Design review of the part built by this model. Coordinates are the model's own, in mm. Face numbers are marked on the shaded views. A direction names the side the tool comes from. Coordinates: 2 decimals unless noted, no trailing zeros. Order: outer loops, then holes, each group sorted by start corner. A loop starts at its lowest first (then second) coordinate and runs counter-clockwise, first axis right, second up. Notation, with made-up numbers: (30, 65.25) -> (87, 65.25) arc R17 ccw to (87, 75.25) -> close; hole circle Ø3 at (5.25, -36.75). An arc over 180 degrees is marked (long way). Write item = value, one per line.
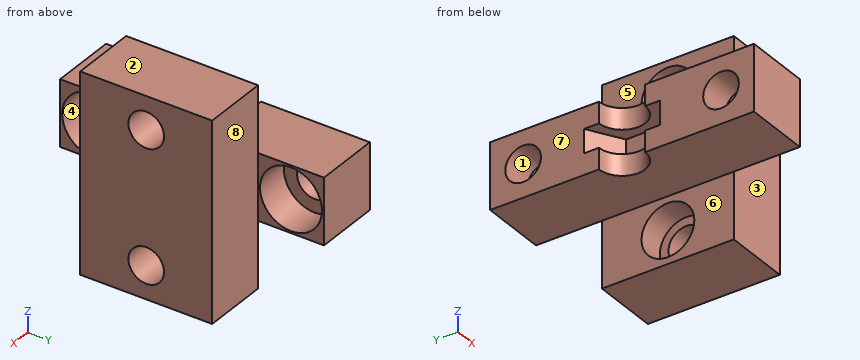
Autodesk Inventor part; units mm, degrees
ref_plane "YZ Plane" through (0, 0, 0) normal (1, 0, 0) x (0, 1, 0)
ref_plane "XZ Plane" through (0, 0, 0) normal (0, 1, 0) x (-1, 0, 0)
ref_plane "XY Plane" through (0, 0, 0) normal (0, 0, 1) x (1, 0, 0)
sketch "Sketch1" plane through (0, 0, 0) normal (0, 0, 1) x (1, 0, 0)
  line L0 (10, -10) -> (-10, -10)
  line L1 (-10, -10) -> (-10, 10)
  line L2 (-10, 10) -> (10, 10)
  line L3 (10, 10) -> (10, -10)
  line L4 (10, -10) -> (-10, 10) construction
  line L5 (-10, -10) -> (10, 10) construction
  line L6 (10, -10) -> (6, -10)
  line L7 (6, 10) -> (10, 10)
  line L8 (10, 10) -> (10, -10)
  line L9 (0, 10) -> (0, -10)
  line L10 (0, -10) -> (0, 10)
  point P0 (0, 0)
  dimension "d0" = 20
  dimension "d1" = 20
extrude "Extrusion1" add sketch "Sketch1" along normal blind 5 contours L0 L9 L2 L3
ref_plane "Work Plane1" through (0, 0, 2.5) normal (0, 0, 1) x (1, 0, 0)
sketch "Sketch2" plane through (0, 0, 2.5) normal (0, 0, 1) x (1, 0, 0)
  line L0 (0, 10) -> (0, -10)
  line L1 (0, 2.8868) -> (2.5, 1.4434)
  line L2 (2.5, 1.4434) -> (2.5, -1.4434)
  line L3 (2.5, -1.4434) -> (0, -2.8868)
  line L4 (0, -2.8868) -> (-2.5, -1.4434)
  line L5 (-2.5, -1.4434) -> (-2.5, 1.4434)
  line L6 (-2.5, 1.4434) -> (0, 2.8868)
  point P0 (0, 0)
  point P1 (0, 0)
  dimension "d12" = 5
extrude "Extrusion2" cut sketch "Sketch2" along normal mid plane 1.8
sketch "Sketch3" plane through (0, 0, 5) normal (0, 0, 1) x (1, 0, 0)
  circle A0 centre (0, 0) radius 1.75
  dimension "d15" = 3.5
extrude "Extrusion3" cut sketch "Sketch3" against normal blind 8
sketch "Sketch4" plane through (10, -10, 0) normal (1, 0, 0) x (0, 0, -1)
  circle A0 centre (-2.5, 17.5) radius 1.35
  circle A1 centre (-2.5, 2.5) radius 1.35
  line L0 (0, 20) -> (-5, 20)
  line L1 (0, 0) -> (-5, 0)
  line L2 (0, 0) -> (0, 20)
  point P0 (0, 10)
  dimension "d18" = 2.5
  dimension "d19" = 2.5
  dimension "d20" = 2.5
  dimension "d21" = 2.5
  dimension "d22" = 2.7
  dimension "d23" = 2.7
extrude "Extrusion4" cut sketch "Sketch4" against normal blind 25
sketch "Sketch5" plane through (10, -10, 0) normal (1, 0, 0) x (0, 0, -1)
  circle A0 centre (-2.5, 17.5) radius 1.35
  circle A1 centre (-2.5, 17.5) radius 2
  circle A2 centre (-2.5, 2.5) radius 1.35
  circle A3 centre (-2.5, 2.5) radius 2
  point P0 (0, 10)
  dimension "d26" = 4
  dimension "d27" = 4
extrude "Extrusion5" cut sketch "Sketch5" against normal blind 4 contours A0 | A1 | A2 | A3
sketch "Sketch6" plane through (0, 0, 5) normal (0, 0, 1) x (1, 0, 0)
  point P0 (0, 0)
sketch "Sketch7" plane through (0, 0, 5) normal (0, 0, 1) x (1, 0, 0)
  line L0 (10, -10) -> (10, 10)
  line L1 (10, 10) -> (5, 10)
  line L2 (5, 10) -> (5, 5)
  line L3 (5, 5) -> (10, 5)
  line L4 (10, 5) -> (10, 10)
  line L5 (0, -10) -> (10, -10)
  line L6 (10, -10) -> (5, -10)
  line L7 (5, -10) -> (5, -5)
  line L8 (5, -5) -> (10, -5)
  line L9 (10, -5) -> (10, -10)
  point P0 (0, 0)
  dimension "d30" = 5
  dimension "d31" = 5
  dimension "d32" = 5
  dimension "d33" = 5
extrude "Extrusion6" cut sketch "Sketch7" against normal blind 10
sketch "Sketch8" plane through (10, -5, 0) normal (1, 0, 0) x (0, 0, -1)
  line L0 (0, 0) -> (5, 0)
  line L1 (5, 0) -> (5, 10)
  line L2 (5, 10) -> (0, 10)
  line L3 (0, 10) -> (0, 0)
  line L4 (-5, 0) -> (-5, 10)
  line L5 (-5, 10) -> (-10, 10)
  line L6 (-10, 10) -> (-10, 0)
  line L7 (-10, 0) -> (-5, 0)
  line L8 (-5, 0) -> (-5, 10)
  circle A0 centre (-7.5, 5) radius 1.35
  circle A1 centre (2.5, 5) radius 1.35
  point P0 (0, 5)
  point P1 (-7.5, 0)
  dimension "d36" = 5
  dimension "d37" = 5
  dimension "d38" = 5
  dimension "d39" = 2.7
  dimension "d40" = 2.7
  dimension "d41" = 5
  dimension "d42" = 5
  dimension "d43" = 5
  dimension "d44" = 5
  dimension "d45" = 2.5
  dimension "d46" = 2.5
extrude "Extrusion7" add sketch "Sketch8" against normal blind 5
sketch "Sketch9" plane through (5, -5, 0) normal (-1, 0, 0) x (0, 0, 1)
  circle A0 centre (7.5, 5) radius 1.35
  circle A1 centre (7.5, 5) radius 2
  circle A2 centre (-2.5, 5) radius 1.35
  circle A3 centre (-2.5, 5) radius 2
  point P0 (0, 5)
  dimension "d49" = 4
  dimension "d50" = 4
extrude "Extrusion8" cut sketch "Sketch9" against normal blind 2 contours A0 | A1 | A2 | A3
sketch "Sketch10" plane through (5, 10, 5) normal (1, 0, 0) x (0, 0, -1)
  circle A0 centre (2.5, -2.5) radius 1.35
  circle A1 centre (2.5, -2.5) radius 2.35
  circle A2 centre (2.5, -17.5) radius 1.35
  circle A3 centre (2.5, -17.5) radius 2.35
  point P0 (5, -10)
  dimension "d53" = 4.7
  dimension "d54" = 4.7
extrude "Extrusion9" cut sketch "Sketch10" against normal blind 2.6
equation "\"d18\" = d19"
equation "\"d20\" = d19"
equation "\"d21\" = d19"
equation "\"d23\" = d22"
equation "\"d27\" = d26"
equation "\"d39\" = d40"
equation "\"d42\" = d41"
equation "\"d50\" = d49"
properties part number "POMSliderMotor"
(1) We need section A-A (y = 0). Write out the cut boundary in (x, z), and give its area (3 significant figures).
Report:
outline = (1.75, 0) -> (5, 0) -> (5, -0.5) -> (7, -0.5) -> (7, -1.15) -> (10, -1.15) -> (10, 6.15) -> (7, 6.15) -> (7, 5.5) -> (5, 5.5) -> (5, 5) -> (1.75, 5) -> (1.75, 3.4) -> (2.5, 3.4) -> (2.5, 1.6) -> (1.75, 1.6) -> close; (5, -5) -> (10, -5) -> (10, -3.85) -> (7, -3.85) -> (7, -4.5) -> (5, -4.5) -> close; (5, 9.5) -> (7, 9.5) -> (7, 8.85) -> (10, 8.85) -> (10, 10) -> (5, 10) -> close
area = 57.7 mm²
(2) We need section D-D (y = 7.5). Write out the cut boundary in (x, z), and give its area (3 significant figures).
Report:
outline = (0, 0) -> (5, 0) -> (5, 0.15) -> (2.4, 0.15) -> (2.4, 1.15) -> (0, 1.15) -> close; (0, 3.85) -> (2.4, 3.85) -> (2.4, 4.85) -> (5, 4.85) -> (5, 5) -> (0, 5) -> close
area = 6.30 mm²
(3) For the marked faces 4, 5, 6, 7 and 8, list the 3-axis set-ups (+Z, -Z, +X, -X, +Y, -Y) from which the entire face can be reached by the end or side of a thin tool; tool diameter is ignored.
Report:
face_4 = +X
face_5 = +Z, -X, +Y, -Y
face_6 = -Z, -X, +Y, -Y
face_7 = +Z, -Z, -X, +Y, -Y
face_8 = +Z, -Z, +X, +Y
(4) We need section C-C (z = -2.5). Write out the cut boundary in (x, y).
Report:
outline = (5, -5) -> (10, -5) -> (10, -1.35) -> (7, -1.35) -> (7, -2) -> (5, -2) -> close; (5, 2) -> (7, 2) -> (7, 1.35) -> (10, 1.35) -> (10, 5) -> (5, 5) -> close
(5) Insertion check: pin 1 (3.5 mm diameter, centred on y = 0, z = 7.5, fed in from -X); pin 2 (3.5 mm diameter, centred on y = 7.5, z = 2.5, fed in from +X); pin 3 (5 mm diameter, centred on y = 8.5, z = 3, fed in from +X). Each pin has a flat end and moves straight along its axis. Give the tip position at first contact, or say it passes through.
Report:
pin_1 = 7
pin_2 = 2.4
pin_3 = 5
(6) For L1, parallel to Y at x = 3.95, z = 2.5; L2, parallel to Y at x = 9.35, z = 7.5; L3, parallel to Y at x = 1.15, z = 2.5, list the stretches that pass through material, from the lowest coordinate up.
Report:
L1 = -10 to -9.85, -5.15 to 5.15, 9.85 to 10
L2 = -5 to -1.35, 1.35 to 5
L3 = -10 to -8.85, -6.15 to -2.22, 2.22 to 6.15, 8.85 to 10
(7) We need section B-B (x = 0.75). Write out the cut boundary in (y, z).
Report:
outline = (-10, 0) -> (-1.58, 0) -> (-1.58, 1.6) -> (-2.45, 1.6) -> (-2.45, 3.4) -> (-1.58, 3.4) -> (-1.58, 5) -> (-10, 5) -> close; (1.58, 0) -> (10, 0) -> (10, 5) -> (1.58, 5) -> (1.58, 3.4) -> (2.45, 3.4) -> (2.45, 1.6) -> (1.58, 1.6) -> close; hole circle Ø2.7 at (-7.5, 2.5); hole circle Ø2.7 at (7.5, 2.5)
(8) The part is to be moulded in two halves that separate along Y. For the marked faces 1, 2 and 3, say which applies: released by +Y, released by -Y, zero draft, split by the parting line, or undercut.
Report:
face_1 = undercut
face_2 = zero draft
face_3 = released by -Y
